Input: part model. Units: mm. Frame: model coordinates. Face numbers are marked on the shaded views. Coordinates: 2 decimals unless noted, no trailing zeros. Order: outer loops, then holes, each group sorted by start corner. A loop starts at its lowest first (then second) coordinate and runs counter-clockwise, first axis right, second up. Notation, with made-up numbers: (60, -23.75) - (76, -23.75) arc R28 cw to (76, 10.25) - close; hole circle Ø9 at (89.25, 12). An arc over 180 degrees is marked (long way). Answer as CSV lines item,"result". Start each with the question number.
Item 1: Section A-A (y = 14.25). Output: boundary loops of the cut face in (x, z).
Item 2: First-contact query: pin 1 (12 mm diameter, centred on x = 69.5, y = 18.5, fed in from -Z); pin 2 (1.5 mm diameter, centred on x = 92, y = 7, fed in from +Z); pin 3 (3 mm diameter, centred on y = 8.5, z = -124.5, fed in from +X). Flat tips, straight axial feed; report the tip coordinate or a pass-through.
Item 3: Section B-B (z = -97.5). Output: boundary loops of the cut face in (x, y), and give its area (3 significant figures).
Item 4: Material intervals for line 1 along Z through (x, y) = (91.5, 3); line 2 along X through (y, z) = (4, -36); line 3 along X through (y, z) = (19, -122), sorted ascending.
Item 5: Draft query along X for the marked faces 1, 2 and 3. Return one class per face: +X half, -X half, draft (parallel to the pull), parting line (faces both ways), or undercut.
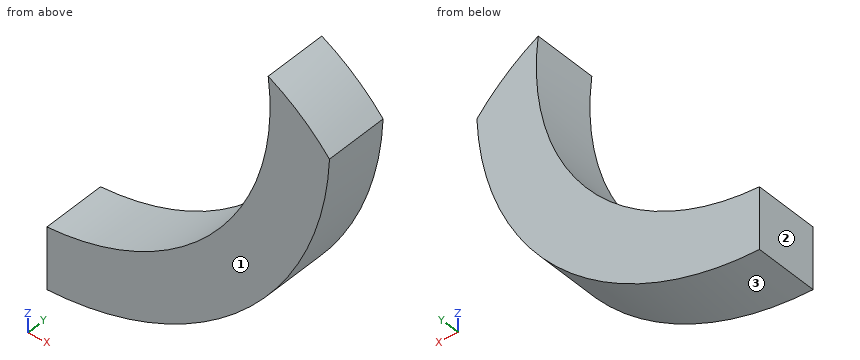
from build123d import *

# Parameters (mm, degrees)
BOSS_EXTRUDE1_DEPTH     = 25.4
BOSS_EXTRUDE1_2_DEPTH   = 25.4
CUT_EXTRUDE1_DEPTH      = 281.867791968
CUT_EXTRUDE1_DEPTH_BACK = 281.867791968
SKETCH2_W               = 46.910236734
SKETCH2_H               = 46.937556504
CUT_EXTRUDE2_DEPTH      = 281.278275978
CUT_EXTRUDE2_DEPTH_BACK = 281.278275978
SKETCH3_OUTSIDE_W       = 231.024
SKETCH3_OUTSIDE_H       = 277.081


with BuildPart() as part:
    # Sketch1 → Boss-Extrude1 (new body)
    with BuildSketch(Plane(origin=(0, 0, 0), x_dir=(1, 0, 0), z_dir=(0, 1, 0))):
        with BuildLine():
            Line((0, 80.02759766), (0, 219.067642019))
            Line((0, 219.067642019), (103.040086398, 219.067642019))
            Line((103.040086398, 219.067642019), (103.040086398, 195.999460881))
            Line((103.040086398, 195.999460881), (23.011829096, 195.999460881))
            Line((23.011829096, 195.999460881), (23.011829096, 161.013213822))
            ThreePointArc((23.011829096, 161.013213822), (101.985495584, 126.901824422), (136.744902109, 48.211224327))
            ThreePointArc((136.744902109, 48.211224327), (146.280346481, 62.911008862), (150.026111113, 80.02759766))
            Line((150.026111113, 80.02759766), (150.026111113, 148.011746996))
            Line((150.026111113, 148.011746996), (172.974333949, 148.011746996))
            Line((172.974333949, 148.011746996), (172.974333949, 80.02759766))
            ThreePointArc((172.974333949, 80.02759766), (86.487166974, 0.037389651), (0, 80.02759766))
        make_face()
        with BuildLine():
            Line((23.011829096, 136.058182002), (23.011829096, 80.02759766))
            ThreePointArc((23.011829096, 80.02759766), (54.48283159, 31.69310754), (112.066438029, 28.410547154))
            ThreePointArc((112.066438029, 28.410547154), (90.841729512, 101.512108787), (23.011829096, 136.058182002))
        make_face(mode=Mode.SUBTRACT)
    extrude(amount=BOSS_EXTRUDE1_DEPTH)

    # Sketch3 outside → Cut-Extrude2 (cut, two sides: drawn at the far end of the back side and taken through both)
    with BuildSketch(Plane(origin=(0, 25.4, 0), x_dir=(1, 0, 0), z_dir=(0, 1, 0)).offset(-CUT_EXTRUDE2_DEPTH_BACK)):
        with Locations((86.487, 109.5525)):
            Rectangle(SKETCH3_OUTSIDE_W, SKETCH3_OUTSIDE_H)
        with BuildLine():
            Line((23.011829096, 161.013213822), (23.011829096, 136.058182002))
            ThreePointArc((23.011829096, 136.058182002), (90.841729512, 101.512108787), (112.066438029, 28.410547154))
            ThreePointArc((112.066438029, 28.410547154), (125.345033884, 37.140114864), (136.744902109, 48.211224327))
            ThreePointArc((136.744902109, 48.211224327), (101.985495584, 126.901824422), (23.011829096, 161.013213822))
        make_face(mode=Mode.SUBTRACT)
    extrude(amount=CUT_EXTRUDE2_DEPTH + CUT_EXTRUDE2_DEPTH_BACK, mode=Mode.SUBTRACT)


with BuildPart() as body_2:
    # Sketch1 → Boss-Extrude1 2 (new body)
    with BuildSketch(Plane(origin=(0, 0, 0), x_dir=(1, 0, 0), z_dir=(0, 1, 0))):
        Polygon((173.927929859, 172.130085515), (150.026111113, 172.130085515), (150.026111113, 195.999460881), (127.017693125, 195.999460881), (127.017693125, 219.067642019), (173.927929859, 219.067642019), align=None)
    extrude(amount=BOSS_EXTRUDE1_2_DEPTH)

    # Sketch2 → Cut-Extrude1 (cut, two sides: drawn at the far end of the back side and taken through both)
    with BuildSketch(Plane(origin=(0, 25.4, 0), x_dir=(1, 0, 0), z_dir=(0, 1, 0)).offset(-CUT_EXTRUDE1_DEPTH_BACK)):
        with Locations((150.472811492, 195.598863767)):
            Rectangle(SKETCH2_W, SKETCH2_H)
    extrude(amount=CUT_EXTRUDE1_DEPTH + CUT_EXTRUDE1_DEPTH_BACK, mode=Mode.SUBTRACT)


solid = part.part
Determined:
1,outline,"(23.01, -161.01) arc R117.87 ccw to (136.74, -48.21) arc R84.12 ccw to (112.07, -28.41) arc R95.8 cw to (23.01, -136.06) - close"
2,pin 1,"stops at z = -152.35"
2,pin 2,"stops at z = -99.13"
2,pin 3,"stops at x = 105.74"
3,outline,"(93.98, 0) - (123.61, 0) - (123.61, 25.4) - (93.98, 25.4) - close"
3,area,"752 mm^2"
4,line 1,"z = -136.14 to -100.71"
4,line 2,"x = 112.72 to 123.89"
4,line 3,"x = 67.29 to 106.65"
5,face 1,"draft"
5,face 2,"-X half"
5,face 3,"+X half"
